```python
from build123d import *

# Parameters (mm, degrees)
SKETCH1_R           = 8.75
BOSS_EXTRUDE1_DEPTH = 4.8
SKETCH2_R           = 3
CUT_EXTRUDE1_DEPTH  = 3
SKETCH3_R           = 2.5
CUT_EXTRUDE2_DEPTH  = 2.5
SKETCH4_R           = 1.375
CUT_EXTRUDE3_DEPTH  = 2.5
CHAMFER1_SIZE       = 2.921


with BuildPart() as part:
    # Sketch1 → Boss-Extrude1 (new body)
    with BuildSketch(Plane(origin=(0, 0, 0), x_dir=(1, 0, 0), z_dir=(0, 1, 0))):
        with Locations(Location((0, 0, 0), (0, 0, 270))):
            Circle(SKETCH1_R)
    extrude(amount=BOSS_EXTRUDE1_DEPTH)

    # Sketch2 → Cut-Extrude1 (cut)
    with BuildSketch(Plane(origin=(0, 4.8, 0), x_dir=(1, 0, 0), z_dir=(0, 1, 0))):
        with Locations(Location((0, 0, 0), (0, 0, 270))):
            Circle(SKETCH2_R)
    extrude(amount=-CUT_EXTRUDE1_DEPTH, mode=Mode.SUBTRACT)

    # Sketch3 → Cut-Extrude2 (cut)
    with BuildSketch(Plane(origin=(0, 4.8, 0), x_dir=(1, 0, 0), z_dir=(0, 1, 0))):
        with Locations(Location((-5.7, 0, 0), (0, 0, 270))):
            Circle(SKETCH3_R)
        with Locations(Location((0, 5.7, 0), (0, 0, 270))):
            Circle(SKETCH3_R)
        with Locations(Location((5.7, 0, 0), (0, 0, 270))):
            Circle(SKETCH3_R)
        with Locations(Location((0, -5.7, 0), (0, 0, 270))):
            Circle(SKETCH3_R)
    extrude(amount=-CUT_EXTRUDE2_DEPTH, mode=Mode.SUBTRACT)

    # Sketch4 → Cut-Extrude3 (cut)
    with BuildSketch(Plane(origin=(0, 2.3, 0), x_dir=(1, 0, 0), z_dir=(0, 1, 0))):
        with Locations(Location((-5.7, 0, 0), (0, 0, 270))):
            Circle(SKETCH4_R)
        with Locations(Location((0, 5.7, 0), (0, 0, 270))):
            Circle(SKETCH4_R)
        with Locations(Location((5.7, 0, 0), (0, 0, 270))):
            Circle(SKETCH4_R)
        with Locations(Location((0, -5.7, 0), (0, 0, 270))):
            Circle(SKETCH4_R)
    extrude(amount=-CUT_EXTRUDE3_DEPTH, mode=Mode.SUBTRACT)

    # Chamfer1
    # the kernel refuses this chamfer: 2.921 mm, written as the material it takes off along each edge
    with BuildSketch(Plane(origin=(0, 4.8, 0), x_dir=(0, 0, 1), z_dir=(-1, 0, 0))) as chamfer1_piece_1:
        Polygon((8.75, -CHAMFER1_SIZE), (8.75 - CHAMFER1_SIZE, 0), (8.75, 0), align=None)
    revolve(axis=Axis((0, 4.8, 0), (0, 1, 0)), mode=Mode.SUBTRACT)


solid = part.part
```
Design review of the part built by this model. Coordinates are the model's own, in mm. A direction names the side the tool comes from. Give positions to 0.01 mm unless a question says otherwise; leave off trailing zeros. Loops run counter-clockwise (first coordinate to the right, second up) from the corner with the lowest first, then second, coordinate; pieces in that order, holes last. Notation, with made-up numbers: (18, -3) -> (49, -3) arc R32 cw to (49, 35) -> close; hole circle Ø5 at (-29, -15). An arc over 180 degrees is marked (long way). Write each question's results on one line, items separated by ' | '.
Q1. Take a section at C-C, the plane z = 0. Write out the cut boundary in (x, y) (3 decimals), plus the area to 3 significant figures.
Reply:
outline: (-8.75, 0) -> (-7.075, 0) -> (-7.075, 2.3) -> (-8.2, 2.3) -> (-8.2, 2.429) -> (-8.75, 1.879) -> close; (-4.325, 0) -> (4.325, 0) -> (4.325, 2.3) -> (3.2, 2.3) -> (3.2, 4.8) -> (3, 4.8) -> (3, 1.8) -> (-3, 1.8) -> (-3, 4.8) -> (-3.2, 4.8) -> (-3.2, 2.3) -> (-4.325, 2.3) -> close; (7.075, 0) -> (8.75, 0) -> (8.75, 1.879) -> (8.2, 2.429) -> (8.2, 2.3) -> (7.075, 2.3) -> close | area: 25.4 mm²
Q2. Take a section at D-D, the plane y = 2.95. Write out the cut boundary in (x, z).
Reply:
outline: (-7.47, -1.76) arc R7.68 ccw to (-1.76, -7.47) arc R2.5 cw (long way) to (1.76, -7.47) arc R7.68 ccw to (7.47, -1.76) arc R2.5 cw (long way) to (7.47, 1.76) arc R7.68 ccw to (1.76, 7.47) arc R2.5 cw (long way) to (-1.76, 7.47) arc R7.68 ccw to (-7.47, 1.76) arc R2.5 cw (long way) to start; hole circle Ø6 at (0, 0)
Q3. Take a section at B-B, the plane y = 1.25. Write out the cut boundary in (x, z) (3 decimals).
Reply:
outline: circle Ø17.5 at (0, 0); hole circle Ø2.75 at (-5.7, 0); hole circle Ø2.75 at (0, -5.7); hole circle Ø2.75 at (0, 5.7); hole circle Ø2.75 at (5.7, 0)
Q4. Machinability: for faces 4 (the face through (0.1, 3.3, 3.2)), 5 (the face through (-3, 4.8, 2)), which of the approach directions +Z, -Z, +X, -X, +Y, -Y give a long, thin tool a straight path to every point of the face, cutting with its end or side? Answer none if there is none.
Reply:
face 4: +Y | face 5: +Z, -Z, +X, -X, +Y
Q5. For pin 1 Ø3 at (x, z) = (-5.7, 0) entering from +Y, flat-tipped, find the tip position at first contact; note if it passes through.
Reply:
pin 1: stops at y = 2.3
Q6. Wall thickness on L1, parallel to X at y = 3.55, z = 0; L2, parallel to Y at x = -6.25, z = -1.5; L3, parallel to X at y = 2.6, z = 4.5: over which ranges is each line inside the solid? List them lowest first.
Reply:
L1: x = -3.2 to -3, 3 to 3.2 | L2: y = 0 to 2.3 | L3: x = -6.65 to -2.19, 2.19 to 6.65
Q7. The part is to be moulded in two halves that separate along X. For faces 1 (the face through (0, 0, 0)), 2 (the face through (-5.297, 4.658, 2.755)), 3 (the face through (4.6, 2.3, 1.1)), say which applies: +X half, -X half, draft (parallel to the pull), parting line (faces both ways), or undercut.
Reply:
face 1: draft | face 2: parting line | face 3: undercut
Q8. Take a section at A-A, the plane x = 0. Write out the cut boundary in (y, z) (3 decimals).
Reply:
outline: (0, -8.75) -> (1.879, -8.75) -> (2.429, -8.2) -> (2.3, -8.2) -> (2.3, -7.075) -> (0, -7.075) -> close; (0, -4.325) -> (2.3, -4.325) -> (2.3, -3.2) -> (4.8, -3.2) -> (4.8, -3) -> (1.8, -3) -> (1.8, 3) -> (4.8, 3) -> (4.8, 3.2) -> (2.3, 3.2) -> (2.3, 4.325) -> (0, 4.325) -> close; (0, 7.075) -> (2.3, 7.075) -> (2.3, 8.2) -> (2.429, 8.2) -> (1.879, 8.75) -> (0, 8.75) -> close
